Here's how the part is built. I have some questions about the finished solid (model axes, mm). A direction names the side the tool comes from. Coordinates: 2 decimals unless noted, no trailing zeros. Write each loop counter-clockwise with the first axis right and the second up, starting at its lowest first coordinate (ties: lowest second). Pieces come first, ordered by that corner, then holes. Notation, with made-up numbers: M 82.5,29 L 113.5,29 A22 cw 113.5,66 Z; hole C 3.5,39 d2. An arc over 180 degrees is marked long. Use a Markdown table: item, result.
```python
from build123d import *

# Parameters (mm, degrees)
F1_DEPTH = 307.975
F2_R     = 14.2875
F3_DEPTH = 25.4
F4_D     = 6.7564
F4_DEPTH = 76.2
F4_TIP   = 2.0298273432


with BuildPart() as f1:
    # F0 (on Front) → F1 (new body)
    with BuildSketch(Plane.XZ):
        Polygon((-41.1849285887, 22.8587505986), (-44.3599285887, 22.8587505986), (-44.3599285887, -2.5412494014), (6.4400714113, -2.5412494014), (6.4400714113, 22.8587505986), (3.2650714113, 22.8587505986), (3.2650714113, 0.6337505986), (-41.1849285887, 0.6337505986), align=None)
    extrude(amount=F1_DEPTH)

    # F2 (on face) → F3 (cut)
    with BuildSketch(Plane(origin=(0, 0, -2.5412494014), x_dir=(1, 0, 0), z_dir=(0, 0, -1))):
        with Locations((-18.9599285887, 280.9875)):
            Circle(F2_R)
        with Locations((-18.9599285887, 26.9875)):
            Circle(F2_R)
    extrude(amount=-F3_DEPTH, mode=Mode.SUBTRACT)

    # F4
    with Locations(Plane(origin=(0, 0, -2.5412494014), x_dir=(1, 0, 0), z_dir=(0, 0, -1))):
        with Locations((-18.9599285887, 217.4875), (-18.9599285887, 115.8875)):
            Hole(F4_D / 2, depth=F4_DEPTH)
            with Locations((0, 0, -(F4_DEPTH + F4_TIP / 2))):  # 118° drill point
                Cone(0, F4_D / 2, F4_TIP, mode=Mode.SUBTRACT)


solid = f1.part
```
1. Will this pin go through, and if not, where does the flat tip stop? pin 1 Ø10 at (x, z) = (-10.5, 8) entering from -Y.
Answers follow:
| item | result |
|---|---|
| pin 1 | passes through |
2. We'd pull the mould along Y, two halves only. Please class faces 3 (the face through (-17, 0, 0)), 4 (the face through (-12.37, -268.31, -0.98)), 5 (the face through (-41.185, -152, 12)), 6 (the face through (-5.332, -31.279, -0.976)): +Y half, -Y half, draft (parallel to the pull), parting line (faces both ways), or undercut.
Answers follow:
| item | result |
|---|---|
| face 3 | +Y half |
| face 4 | undercut |
| face 5 | draft |
| face 6 | undercut |
3. Suppose I cut it at B-B on y = -205.5. Write out the boundary of the cut face in (x, z).
Answers follow:
| item | result |
|---|---|
| outline | M -44.36,-2.54 L 6.44,-2.54 L 6.44,22.86 L 3.27,22.86 L 3.27,0.63 L -41.18,0.63 L -41.18,22.86 L -44.36,22.86 Z |
4. Suppose I cut it at D-D on y = -278. Write out the boundary of the cut face in (x, z), and give its area (3 significant figures).
Answers follow:
| item | result |
|---|---|
| outline | M -44.36,-2.54 L -32.93,-2.54 L -32.93,0.63 L -41.18,0.63 L -41.18,22.86 L -44.36,22.86 Z; M -4.99,-2.54 L 6.44,-2.54 L 6.44,22.86 L 3.27,22.86 L 3.27,0.63 L -4.99,0.63 Z |
| area | 214 mm2 |
5. I need wall thicknesses on probe 1 along X at (y, z) = (-295, 19.25); probe 2 along Z at (x, y) = (-5.5, -275). Which ranges of each line are inside material? Lowest first, please.
Answers follow:
| item | result |
|---|---|
| probe 1 | x = -44.36 to -41.18, 3.27 to 6.44 |
| probe 2 | z = -2.54 to 0.63 |
6. Which directions (+Z, -Z, +X, -X, +Y, -Y) give clear straight access to the entire face, cutting with the end or side of a thin tool? Please do faces 1 (the face through (-17, -307.975, 0)), 2 (the face through (3.265, -152, 12)).
Answers follow:
| item | result |
|---|---|
| face 1 | +Z, -Z, +X, -X, -Y |
| face 2 | +Z, +Y, -Y |
7. Suppose I cut it at C-C on x = -8. Write out the boundary of the cut face in (y, z) (3 decimals).
Answers follow:
| item | result |
|---|---|
| outline | M -307.975,-2.541 L -290.153,-2.541 L -290.153,0.634 L -307.975,0.634 Z; M -271.822,-2.541 L -36.153,-2.541 L -36.153,0.634 L -271.822,0.634 Z; M -17.822,-2.541 L 0,-2.541 L 0,0.634 L -17.822,0.634 Z |
8. Suppose I cut it at A-A on z = 14.5. Write out the boundary of the cut face in (x, y) (3 decimals), and give its area (3 significant figures).
Answers follow:
| item | result |
|---|---|
| outline | M -44.36,-307.975 L -41.185,-307.975 L -41.185,0 L -44.36,0 Z; M 3.265,-307.975 L 6.44,-307.975 L 6.44,0 L 3.265,0 Z |
| area | 1,960 mm2 |
